```python
from build123d import *

# Parameters (mm, degrees)
SKETCH1_R                           = 17.5
SKETCH1_R_2                         = 2.5
BOSS_EXTRUDE1_DEPTH                 = 10
BOSS_EXTRUDE2_START                 = 5
SKETCH1_3_R                         = 17.5
BOSS_EXTRUDE2_DEPTH                 = 5
CUT_EXTRUDE1_REACH                  = 32.582
CUT_EXTRUDE1_END_RADIUS             = 17.5
SKETCH8_R                           = 1.5
CUT_EXTRUDE1_DIRECTION_2_REACH      = 32.582
CUT_EXTRUDE1_DIRECTION_2_END_RADIUS = 2.5
CUT_EXTRUDE2_DEPTH                  = 2.2
SKETCH10_W                          = 6.5
SKETCH10_H                          = 6.5
BOSS_EXTRUDE3_DEPTH                 = 14


with BuildPart() as part:
    # Sketch1 → Boss-Extrude1 (new body)
    with BuildSketch(Plane.XY):
        Circle(SKETCH1_R)
        Circle(SKETCH1_R_2, mode=Mode.SUBTRACT)
    extrude(amount=-BOSS_EXTRUDE1_DEPTH)

    # Sketch1<3> → Boss-Extrude2 (add)
    with BuildSketch(Plane.XY.offset(BOSS_EXTRUDE2_START)):
        Circle(SKETCH1_3_R)
    extrude(amount=-BOSS_EXTRUDE2_DEPTH)

    # Cut-Extrude1: up to this cylinder (the profile starts inside it)
    cut_extrude1_end = Plane(origin=(0, 0, -5.7), z_dir=(0, 0, 1)) * Cylinder(CUT_EXTRUDE1_END_RADIUS, 101.164, mode=Mode.PRIVATE)
    # Sketch8 → Cut-Extrude1 (cut, up to the surface)
    with BuildSketch(Plane(origin=(5.5, 0, 0), x_dir=(0, 0, -1), z_dir=(1, 0, 0)), mode=Mode.PRIVATE) as cut_extrude1_sk1:
        with Locations((5.7, 0)):
            Circle(SKETCH8_R)
    cut_extrude1_tool1 = extrude(cut_extrude1_sk1.sketch, amount=CUT_EXTRUDE1_REACH, mode=Mode.PRIVATE) & cut_extrude1_end
    cut_extrude1 = cut_extrude1_tool1.solids().sort_by_distance((5.5, 0, -5.7))[0]
    add(cut_extrude1, mode=Mode.SUBTRACT)

    # Cut-Extrude1 direction 2: up to this cylinder (the profile starts outside it)
    cut_extrude1_direction_2_end = Plane(origin=(0, 0, -5.7), z_dir=(0, 0, 1)) * Cylinder(CUT_EXTRUDE1_DIRECTION_2_END_RADIUS, 71.164, mode=Mode.PRIVATE)
    # Sketch8 → Cut-Extrude1 direction 2 (cut, up to the surface)
    with BuildSketch(Plane(origin=(5.5, 0, 0), x_dir=(0, 0, -1), z_dir=(1, 0, 0)), mode=Mode.PRIVATE) as cut_extrude1_direction_2_sk1:
        with Locations((5.7, 0)):
            Circle(SKETCH8_R)
    cut_extrude1_direction_2_tool1 = extrude(cut_extrude1_direction_2_sk1.sketch, amount=-CUT_EXTRUDE1_DIRECTION_2_REACH, mode=Mode.PRIVATE) - cut_extrude1_direction_2_end
    cut_extrude1_direction_2 = cut_extrude1_direction_2_tool1.solids().sort_by_distance((5.5, 0, -5.7))[0]
    add(cut_extrude1_direction_2, mode=Mode.SUBTRACT)
    cut_extrude1 = cut_extrude1 + cut_extrude1_direction_2  # both directions under the feature's name, for the pattern or mirror that repeats it

    # Sketch8<4> → Cut-Extrude2 (cut)
    with BuildSketch(Plane(origin=(5.5, 0, 0), x_dir=(0, 0, -1), z_dir=(1, 0, 0))):
        Polygon((8.5, 2.8), (2.9, 2.8), (2.9, -2.8), (8.5, -2.8), (10, -2.8), (10, 2.8), align=None)
    cut_extrude2 = extrude(amount=CUT_EXTRUDE2_DEPTH, mode=Mode.SUBTRACT)

    # Mirror1: Cut-Extrude1, Cut-Extrude2 across plane
    add(cut_extrude1.mirror(Plane(origin=(0, 0, 0), x_dir=(0, 0, 1), z_dir=(1, 0, 0))), mode=Mode.SUBTRACT)
    add(cut_extrude2.mirror(Plane(origin=(0, 0, 0), x_dir=(0, 0, 1), z_dir=(1, 0, 0))), mode=Mode.SUBTRACT)

    # Sketch10 → Boss-Extrude3 (add)
    with BuildSketch(Plane.XY.offset(5)):
        Rectangle(SKETCH10_W, SKETCH10_H)
    extrude(amount=BOSS_EXTRUDE3_DEPTH)


solid = part.part
```
CAD build for the part. Positions are in the model's coordinates, mm. A direction names the side the tool comes from. Coordinates: 2 decimals unless noted, no trailing zeros. Write each loop counter-clockwise with the first axis right and the second up, starting at its lowest first coordinate (ties: lowest second). Pieces come first, ordered by that corner, then holes. Notation, with made-up numbers: (34.25, -36) -> (51.25, -36) arc R18 cw to (51.25, -25) -> close; hole circle Ø7 at (-33.5, -26.5). An arc over 180 degrees is marked (long way). Return JSON: item names as keys, results as strings. Group by question number.
Q1. Cut at A-A, the plane z = -5.7. Give the cut face in (x, y), then the cut area to 3 significant figures.
Q2. Cut at C-C, the plane x = 0. Give the cut face in (y, z), then the cut area to 3 significant figures.
Q3. Which spindle directions (+Z, -Z, +X, -X, +Y, -Y) get a long thin tool onto all of the face, cutting with end or side? Do faces 1 (the face through (0, 3.25, 12)), 2 (the face through (3.25, 0, 12)), 3 (the face through (-7, 2.8, -6)). Say none if no direction does.
Q4. Cut at B-B, the plane x = 10.5. Give the cut face in (y, z), then the cut area to 3 significant figures.
Q5. Cut at D-D, the plane z = -2.25. Give the cut face in (x, y), then the cut area to 3 significant figures.
Q6. Flat gauge pins, fed straight in: pin 1 (2 mm diameter, centred on y = 0, z = 9.5, fed in from -X); pin 2 (1.5 mm diameter, centred on x = -8.5, y = 7.5, fed in from +Z); pin 3 (7 mm diameter, centred on y = -0.5, z = 9, fed in from +X); pin 4 (3 mm diameter, centred on y = 1, z = -7, fed in from -X). Where does each tip first touch, or does it go through?
Q7. Pull direction Y, two halves, no side cores. Call faces 4 (the face through (16.166, -6.703, -2.395)), 5 (the face through (0, 0, 19)), 6 (the face through (0, 0, 0)): released by +Y, released by -Y, zero draft, split by the parting line, or undercut.
Q8. Drill centre lines: line 1 (Z direction, x = 4, y = 0); line 2 (Z direction, x = -3.15, y = 0); line 3 (Z direction, x = -8, y = -13). Where is each one in solid material? Low to high.
Returned:
{
 "1": {"outline": "(-17.44, -1.5) arc R17.5 ccw to (17.44, -1.5) -> (7.7, -1.5) -> (7.7, -2.8) -> (5.5, -2.8) -> (5.5, -1.5) -> (2, -1.5) arc R2.5 cw to (-2, -1.5) -> (-5.5, -1.5) -> (-5.5, -2.8) -> (-7.7, -2.8) -> (-7.7, -1.5) -> close; (-17.44, 1.5) -> (-7.7, 1.5) -> (-7.7, 2.8) -> (-5.5, 2.8) -> (-5.5, 1.5) -> (-2, 1.5) arc R2.5 cw to (2, 1.5) -> (5.5, 1.5) -> (5.5, 2.8) -> (7.7, 2.8) -> (7.7, 1.5) -> (17.44, 1.5) arc R17.5 ccw to start", "area": "840 mm2"},
 "2": {"outline": "(-17.5, -10) -> (-2.5, -10) -> (-2.5, 0) -> (2.5, 0) -> (2.5, -10) -> (17.5, -10) -> (17.5, 5) -> (3.25, 5) -> (3.25, 19) -> (-3.25, 19) -> (-3.25, 5) -> (-17.5, 5) -> close", "area": "566 mm2"},
 "3": {"face 1": "+Z, +X, -X, +Y", "face 2": "+Z, +X, +Y, -Y", "face 3": "-Z"},
 "4": {"outline": "(-14, -10) -> (14, -10) -> (14, 5) -> (-14, 5) -> close; hole circle Ø3 at (0, -5.7)", "area": "413 mm2"},
 "5": {"outline": "circle Ø35 at (0, 0); hole circle Ø5 at (0, 0)", "area": "942 mm2"},
 "6": {"pin 1": "stops at x = -3.25", "pin 2": "stops at z = 5", "pin 3": "stops at x = 3.25", "pin 4": "stops at x = -17.5"},
 "7": {"face 4": "split by the parting line", "face 5": "zero draft", "face 6": "undercut"},
 "8": {"line 1": "z = -10 to -7.2, -4.2 to 5", "line 2": "z = -10 to -7.2, -4.2 to 19", "line 3": "z = -10 to 5"}
}
